from build123d import *

# Parameters (mm, degrees)
SKETCH1_R           = 3.175
BOSS_EXTRUDE1_DEPTH = 7.112


with BuildPart() as part:
    # Sketch1 → Boss-Extrude1 (new body)
    with BuildSketch(Plane.XY):
        with BuildLine():
            Line((46.99, 0), (73.66, 0))
            Line((73.66, 0), (73.66, 12.7))
            Line((73.66, 12.7), (0, 12.7))
            Line((0, 12.7), (0, 0))
            Line((0, 0), (26.67, 0))
            ThreePointArc((26.67, 0), (36.83, 5.08), (46.99, 0))
        make_face()
        with Locations((12.7, 6.35)):
            Circle(SKETCH1_R, mode=Mode.SUBTRACT)
        with Locations((60.96, 6.35)):
            Circle(SKETCH1_R, mode=Mode.SUBTRACT)
    extrude(amount=BOSS_EXTRUDE1_DEPTH)


solid = part.part
Source: CAD feature listing. Evaluate the final solid. Frame: model axes, mm. Give positions to 0.01 mm unless a question says otherwise; leave off trailing zeros. Write each loop counter-clockwise with the first axis right and the second up, starting at its lowest first coordinate (ties: lowest second). Pieces come first, ordered by that corner, then holes. Notation, with made-up numbers: M 49.25,-13 L 84.25,-13 A24 cw 84.25,25 Z; hole C 61.25,26 d11. An arc over 180 degrees is marked long. Return JSON: item names as keys, results as strings. Group by question number.
1) Pull-direction query (Y, two-part tool) for faces 1 (the face through (10.36, 8.496, 3.506)), 2 (the face through (37, 12.7, 4)), 3 (the face through (36, 6, 0)); classes: pulls with the +Y half, pulls with the -Y half, needs draft (parallel to the pull), parting line crosses it, or undercut.
2) Cut plane C-C, the plane y = 6.35. Output: boundary loops of the cut face in (x, z) (3 decimals).
3) Material intervals for line 1 along Y through (x, z) = (12.7, 4.75) (3 decimals); line 2 along X through (y, z) = (8.75, 3); line 3 along X through (y, z) = (2.25, 5), sorted ascending. Write a range as [from, to].
4) Cut plane D-D, the plane x = 43. Output: boundary loops of the cut face in (y, z).
5) Cut plane B-B, the plane x = 60.96. Output: boundary loops of the cut face in (y, z) (3 decimals), plus the area to 3 significant figures.
6) Cut plane A-A, the plane z = 2. Output: boundary loops of the cut face in (x, y) (3 decimals).
7) Pin query (flat end, axial travel): P1, Ø2, axis at x = 18, y = 10.5, coming from the -Z side. Return the tip coordinate at first contact, or that it passes through.
Recorded:
{
 "1": {"face 1": "undercut", "face 2": "pulls with the +Y half", "face 3": "needs draft"},
 "2": {"outline": "M 0,0 L 9.525,0 L 9.525,7.112 L 0,7.112 Z; M 15.875,0 L 57.785,0 L 57.785,7.112 L 15.875,7.112 Z; M 64.135,0 L 73.66,0 L 73.66,7.112 L 64.135,7.112 Z"},
 "3": {"line 1": "y = [0, 3.175], [9.525, 12.7]", "line 2": "x = [0, 10.62], [14.78, 58.88], [63.04, 73.66]", "line 3": "x = [0, 28.84], [44.82, 73.66]"},
 "4": {"outline": "M 3.48,0 L 12.7,0 L 12.7,7.11 L 3.48,7.11 Z"},
 "5": {"outline": "M 0,0 L 3.175,0 L 3.175,7.112 L 0,7.112 Z; M 9.525,0 L 12.7,0 L 12.7,7.112 L 9.525,7.112 Z", "area": "45.2 mm²"},
 "6": {"outline": "M 0,0 L 26.67,0 A12.7 cw 46.99,0 L 73.66,0 L 73.66,12.7 L 0,12.7 Z; hole C 12.7,6.35 d6.35; hole C 60.96,6.35 d6.35"},
 "7": {"P1": "stops at z = 0"}
}
